from build123d import *

# Parameters (mm, degrees)
SKETCH_1_R      = 1.6
SKETCH_1_W      = 10
SKETCH_1_H      = 8
EXTRUDE_1_DEPTH = 3


with BuildPart() as part:
    # ｽｹｯﾁ1 → ﾎﾞｽ - 押し出し1 (new body)
    with BuildSketch(Plane(origin=(0, 0, 0), x_dir=(0, 0, -1), z_dir=(1, 0, 0))):
        Polygon((17, 27), (17, 7), (80, 7), (80, 27), (75, 27), (75, 30), (70, 30), (70, 27), (50, 27), (50, 30), (45, 30), (45, 27), align=None)
        with Locations((22, 17)):
            Circle(SKETCH_1_R, mode=Mode.SUBTRACT)
        with Locations((36.14, 21.05)):
            Rectangle(SKETCH_1_W, SKETCH_1_H, mode=Mode.SUBTRACT)
    extrude(amount=EXTRUDE_1_DEPTH)


solid = part.part
Can you work these out from the model? Positions are in its coordinate system, mm. A direction names the side the tool comes from. Give positions to 0.01 mm unless a question says otherwise; leave off trailing zeros. Loops run counter-clockwise (first coordinate to the right, second up) from the corner with the lowest first, then second, coordinate; pieces in that order, holes last. Notation, with made-up numbers: (68.25, 13) - (115.25, 13) arc R23 ccw to (115.25, 33) - close; hole circle Ø4 at (86.25, 16). An arc over 180 degrees is marked (long way). Answer as a JSON object with one key per item and string values.
Q1. Will these pins go through, and if not, where does the flat tip stop? P1, Ø1.5, axis at x = 1, z = -55, coming from the +Y side; P2, Ø1.5, axis at x = 1, y = 28.5, coming from the +Z side.
Geometry says:
{"P1": "y = 27", "P2": "z = -45"}
Q2. Which directions (+Z, -Z, +X, -X, +Y, -Y) give clear straight access to the entire face, cutting with the end or side of a thin tool? Please do faces 1 (the flat face through (1, 28, -50)), 2 (the flat face through (1, 17.05, -36)), 3 (the flat face through (1, 27, -78)), 4 (the flat face through (1, 29, -45)).
Geometry says:
{"face 1": "+X, -X, +Y", "face 2": "+X, -X", "face 3": "-Z, +X, -X, +Y", "face 4": "+Z, +X, -X, +Y"}
Q3. Imagine slicing it at B-B on z = -22. Write out the boundary of the cut face in (x, y), plus the area to 3 significant figures.
Geometry says:
{"outline": "(0, 7) - (3, 7) - (3, 15.4) - (0, 15.4) - close; (0, 18.6) - (3, 18.6) - (3, 27) - (0, 27) - close", "area": "50.4 mm²"}
Q4. Imagine slicing it at C-C on x = 1.7. Write out the boundary of the cut face in (y, z), plus the area to 3 significant figures.
Geometry says:
{"outline": "(7, -80) - (27, -80) - (27, -75) - (30, -75) - (30, -70) - (27, -70) - (27, -50) - (30, -50) - (30, -45) - (27, -45) - (27, -17) - (7, -17) - close; hole circle Ø3.2 at (17, -22); hole (17.05, -41.14) - (25.05, -41.14) - (25.05, -31.14) - (17.05, -31.14) - close", "area": "1,200 mm²"}
Q5. If I drill on L1, parallel to Y at x = 1.8, z = -22; L2, parallel to Z at x = 0.35, y = 24.75; L3, parallel to Y at x = 2.3, z = -64, over which ranges is the centre line in solid material (lowest first)?
Geometry says:
{"L1": "7 to 15.4, 18.6 to 27", "L2": "-80 to -41.14, -31.14 to -17", "L3": "7 to 27"}
Q6. Imagine slicing it at A-A on y = 20.25. Write out the boundary of the cut face in (x, z), plus the area to 3 significant figures.
Geometry says:
{"outline": "(0, -80) - (3, -80) - (3, -41.14) - (0, -41.14) - close; (0, -31.14) - (3, -31.14) - (3, -17) - (0, -17) - close", "area": "159 mm²"}
Q7. If we mould it in two halves opening along Y, with no side actions, what happens to faces 5 (the flat face through (1, 25.05, -36)), 6 (the flat face through (1, 30, -48)), 7 (the flat face through (1, 21, -31.14)), 8 (the flat face through (1, 17, -80))? For each: pulls with the +Y half, pulls with the -Y half, needs draft (parallel to the pull), parting line crosses it, or undercut.
Geometry says:
{"face 5": "undercut", "face 6": "pulls with the +Y half", "face 7": "undercut", "face 8": "needs draft"}
